For this review, take the finished solid that the model builds, in its own axes (mm). Round coordinates to 2 decimals unless told otherwise and drop trailing zeros. Order: outer loops, then holes, each group sorted by start corner. A loop starts at its lowest first (then second) coordinate and runs counter-clockwise, first axis right, second up. Notation, with made-up numbers: M -24.5,63.5 L 2.5,63.5 A27 cw 2.5,83.5 Z; hole C 32,26 d8. An arc over 180 degrees is marked long. Put each result on its own line as item: value.
from build123d import *

# Parameters (mm, degrees)
SKETCH1_R           = 2.6
SKETCH1_R_2         = 3.6
BOSS_EXTRUDE1_DEPTH = 5


with BuildPart() as part:
    # Sketch1 → Boss-Extrude1 (new body)
    with BuildSketch(Plane(origin=(0, 0, 0), x_dir=(1, 0, 0), z_dir=(0, 1, 0))):
        with BuildLine():
            Line((-31.117126255, 8.600085423), (-11.115122128, -30.309917119))
            ThreePointArc((-11.115122128, -30.309917119), (0.002513408, -37.095067694), (11.119596019, -30.309011222))
            Line((11.119596019, -30.309011222), (31.117591892, 8.60099132))
            ThreePointArc((31.117591892, 8.60099132), (30.669449235, 20.827449945), (20, 26.814934838))
            Line((20, 26.814934838), (-20, 26.814934838))
            ThreePointArc((-20, 26.814934838), (-30.669714562, 20.82701524), (-31.117126255, 8.600085423))
        make_face()
        with Locations(Location((-20, 14.314934838, 0), (0, 0, 270))):
            Circle(SKETCH1_R, mode=Mode.SUBTRACT)
        with Locations(Location((20, 14.314934838, 0), (0, 0, 270))):
            Circle(SKETCH1_R, mode=Mode.SUBTRACT)
        with Locations(Location((0.002004127, -24.595067704, 0), (0, 0, 270))):
            Circle(SKETCH1_R_2, mode=Mode.SUBTRACT)
    extrude(amount=BOSS_EXTRUDE1_DEPTH)


solid = part.part
(1) Draft analysis for pull direction Z (two halves, no side actions). For faces 1 (the face through (0.2, 2.5, 21)), 2 (the face through (-30.575, 2.465, -20.979)), 3 (the face through (-19.219, 2.465, -11.835)), 4 (the face through (-0.189, 2.465, 37.094)), state which applies: released by +Z, released by -Z, zero draft, split by the parting line, or undercut.
A:
face 1: undercut
face 2: split by the parting line
face 3: undercut
face 4: released by +Z
(2) To check wall thickness, follow L1, parallel to X at y = 4.5, z = -16; L2, parallel to X at y = 1.2, z = -14; L3, parallel to X at y = 2.5, z = 13. State the ranges of each line that lie inside material, in increasing order.
A:
L1: x = -32.39 to -21.98, -18.02 to 18.02, 21.98 to 32.39
L2: x = -32.5 to -22.58, -17.42 to 17.42, 22.58 to 32.5
L3: x = -20.01 to 20.02
(3) Add section A-A on y = 1.4. Give the boundary of the cut face in (x, z), then the cut area to 3 significant figures.
A:
outline: M -31.12,-8.6 A12.5 ccw -20,-26.81 L 20,-26.81 A12.5 ccw 31.12,-8.6 L 11.12,30.31 A12.5 ccw -11.12,30.31 Z; hole C -20,-14.31 d5.2; hole C 0,24.6 d7.2; hole C 20,-14.31 d5.2
area: 2,780 mm2
(4) Insertion check: pin 1 Ø4 at (x, z) = (20, -14.31) entering from +Y; pin 2 Ø1 at (y, z) = (3, -12) entering from -X. Each pin has a flat end and moves straight along its axis. Give the tip position at first contact, or say it passes through.
A:
pin 1: passes through
pin 2: stops at x = -32.37
(5) Add section B-B on z = 18. Give the boundary of the cut face in (x, y), then the cut area to 3 significant figures.
A:
outline: M -17.44,0 L 17.45,0 L 17.45,5 L -17.44,5 Z
area: 174 mm2
(6) Add section C-C on x = -28. Give the boundary of the cut face in (y, z).
A:
outline: M 0,-23.92 L 5,-23.92 L 5,-2.54 L 0,-2.54 Z
